Input: dimensioned drawing with shaded views. Units: mm. Origin: part minimum x, y, z. A direction names the side the tool comes from. Coordinates: 2 decimals unless noted, no trailing zeros. Order: outer loops, then holes, each group sorted by start corner. A loop starts at its lowest first (then second) coordinate and runs counter-clockwise, first axis right, second up. Notation, with made-up numbers: (48, -15.75) - (66, -15.75) arc R25 cw to (66, 13.25) - close; hole circle Ø8 at (54, 76). An arc over 180 degrees is marked (long way). Answer as CSV lines item,"result". Start each with the question number.
Item 1: Draft query along X for the marked faces 1, 2, 3 and 4. Return one class per face: +X half, -X half, draft (parallel to the pull), parting line (faces both ways), or undercut.
Item 2: Section B-B (y = 5). Output: boundary loops of the cut face in (x, z).
Item 3: Material intervals for line 1 along X through (y, z) = (3.5, 56.5); line 2 along Z through (x, y) = (6, 3.5), sorted ascending.
Item 4: Section A-A (x = 39.55). Output: boundary loops of the cut face in (y, z), and give its area (3 significant figures).
Item 5: Section C-C (z = 59). Output: boundary loops of the cut face in (x, y).
Item 6: Section D-D (x = 19). Output: boundary loops of the cut face in (y, z).
Item 7: First-contact query: pin 1 (1.2 mm diameter, centred on x = 3, y = 4, fed in from +Z); pin 2 (3 mm diameter, centred on x = 2.5, y = 4, fed in from -Z). Flat tips, straight axial feed; report the tip coordinate or a pass-through.
Item 8: Access query for the marked faces 5 and 6. Directions: +Z, -Z, +X, -X, +Y, -Y. A direction counts if a zero-diameter tool reaches every point of the face in a straight line with its end or side. Return the directions, or none.
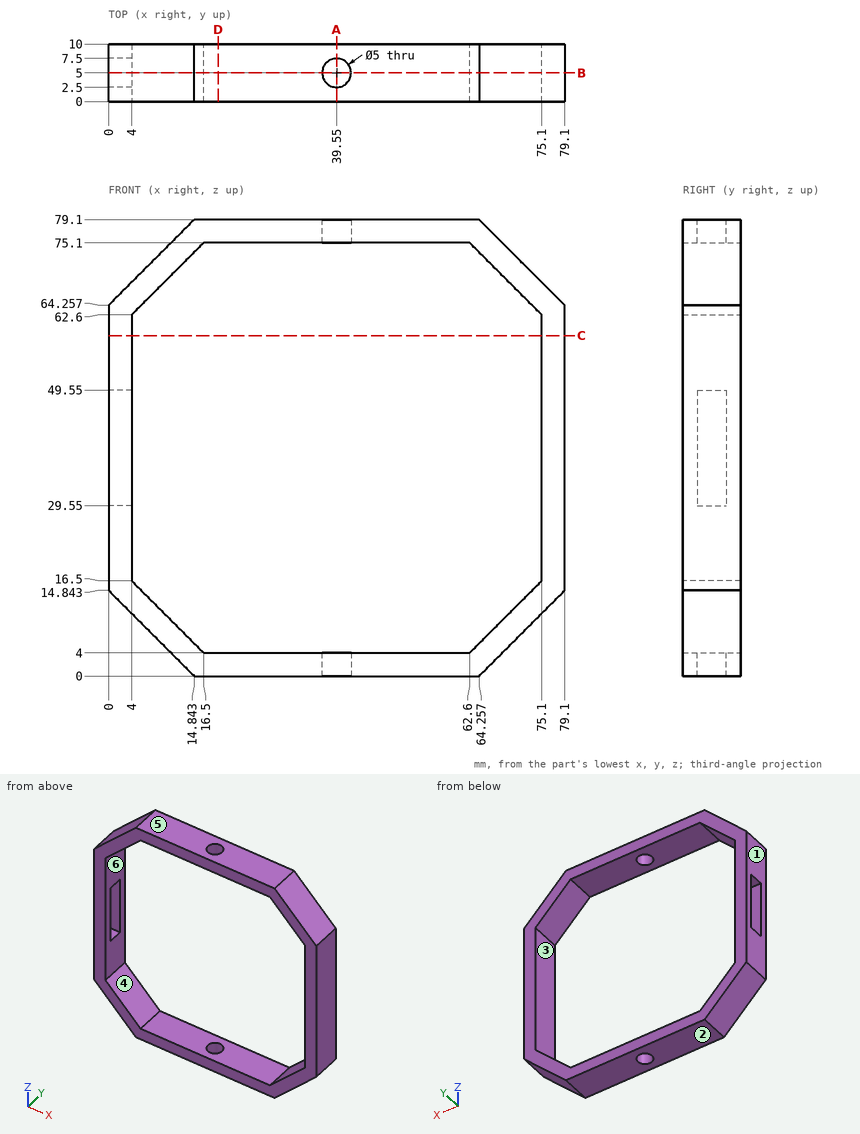
Determined:
1,face 1,"-X half"
1,face 2,"draft"
1,face 3,"undercut"
1,face 4,"undercut"
2,outline,"(0, 14.84) - (14.84, 0) - (37.05, 0) - (37.05, 4) - (16.5, 4) - (4, 16.5) - (4, 29.55) - (0, 29.55) - close; (0, 49.55) - (4, 49.55) - (4, 62.6) - (16.5, 75.1) - (37.05, 75.1) - (37.05, 79.1) - (14.84, 79.1) - (0, 64.26) - close; (42.05, 0) - (64.26, 0) - (79.1, 14.84) - (79.1, 64.26) - (64.26, 79.1) - (42.05, 79.1) - (42.05, 75.1) - (62.6, 75.1) - (75.1, 62.6) - (75.1, 16.5) - (62.6, 4) - (42.05, 4) - close"
3,line 1,"x = 0 to 4, 75.1 to 79.1"
3,line 2,"z = 8.84 to 14.5, 64.6 to 70.26"
4,outline,"(0, 0) - (2.5, 0) - (2.5, 4) - (0, 4) - close; (0, 75.1) - (2.5, 75.1) - (2.5, 79.1) - (0, 79.1) - close; (7.5, 0) - (10, 0) - (10, 4) - (7.5, 4) - close; (7.5, 75.1) - (10, 75.1) - (10, 79.1) - (7.5, 79.1) - close"
4,area,"40.0 mm^2"
5,outline,"(0, 0) - (4, 0) - (4, 10) - (0, 10) - close; (75.1, 0) - (79.1, 0) - (79.1, 10) - (75.1, 10) - close"
6,outline,"(0, 0) - (10, 0) - (10, 4) - (0, 4) - close; (0, 75.1) - (10, 75.1) - (10, 79.1) - (0, 79.1) - close"
7,pin 1,"stops at z = 67.86"
7,pin 2,"stops at z = 10.84"
8,face 5,"+Z, +X, -X, +Y, -Y"
8,face 6,"+Y, -Y"
